from build123d import *

# Parameters (mm, degrees)
SKETCH_1_W          = 57.566503366
SKETCH_1_H          = 9.194649843
EXTRUDE_2_DEPTH     = 9
SKETCH_2_R          = 4.304670881
CUT_EXTRUDE_1_DEPTH = 9
SKETCH_3_R          = 3.25
CUT_EXTRUDE_4_DEPTH = 59.986811199
SKETCH_4_R          = 1.995507564
CUT_EXTRUDE_5_DEPTH = 59.986811199
FILLET_4_R          = 0.2


with BuildPart() as part:
    # 草图1 → 凸台-拉伸2 (new body)
    with BuildSketch(Plane(origin=(0, 0, 0), x_dir=(1, 0, 0), z_dir=(0, 1, 0))):
        with Locations((28.783251683, 4.597324922)):
            Rectangle(SKETCH_1_W, SKETCH_1_H)
    extrude(amount=EXTRUDE_2_DEPTH)

    # 草图2 → 切除-拉伸1 (cut)
    with BuildSketch(Plane(origin=(0, 9, 0), x_dir=(1, 0, 0), z_dir=(0, 1, 0))):
        with Locations(Location((5.562922539, 4.537375707, 0), (0, 0, 270))):
            Circle(SKETCH_2_R)
    extrude(amount=-CUT_EXTRUDE_1_DEPTH, mode=Mode.SUBTRACT)

    # 草图3 → 切除-拉伸4 (cut, through all)
    with BuildSketch(Plane.XY):
        with Locations((25.905689379, 4.639881501)):
            Circle(SKETCH_3_R)
        with Locations((30.901457267, 4.679847644)):
            Circle(SKETCH_3_R)
    extrude(amount=-CUT_EXTRUDE_4_DEPTH, mode=Mode.SUBTRACT)

    # 草图4 → 切除-拉伸5 (cut, through all)
    with BuildSketch(Plane(origin=(0, 9, 0), x_dir=(1, 0, 0), z_dir=(0, 1, 0))):
        with Locations(Location((45.569031787, 4.648915429, 0), (0, 0, 270))):
            Circle(SKETCH_4_R)
        with Locations(Location((53.08266669, 4.648915429, 0), (0, 0, 270))):
            Circle(SKETCH_4_R)
    extrude(amount=-CUT_EXTRUDE_5_DEPTH, mode=Mode.SUBTRACT)

    # 圆角4
    fillet_4_edges = [part.edges().sort_by_distance(p)[0] for p in [
        (5.562922539, 9, -8.842046587),
        (45.569031787, 9, -6.644422993),
        (53.08266669, 9, -6.644422993),
    ]]
    fillet(fillet_4_edges, radius=FILLET_4_R)


solid = part.part
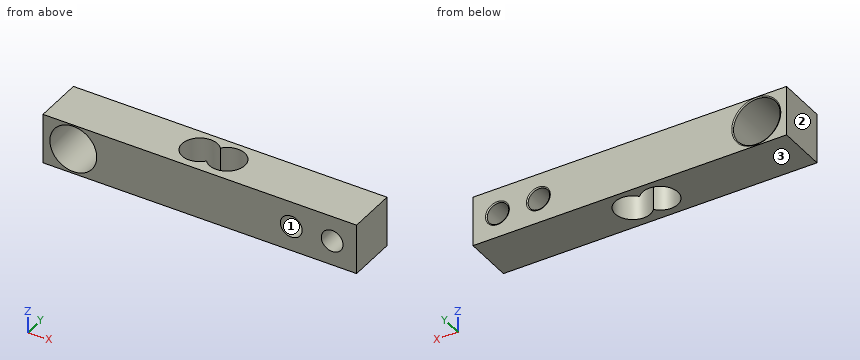
The model under review builds one solid part; all positions refer to its coordinate system, in mm. Face numbers are marked on the shaded views. Coordinates: 2 decimals unless noted, no trailing zeros. Order: outer loops, then holes, each group sorted by start corner. A loop starts at its lowest first (then second) coordinate and runs counter-clockwise, first axis right, second up. Notation, with made-up numbers: (57, 3.25) -> (104, 3.25) arc R13 ccw to (104, 26.25) -> close; hole circle Ø5 at (17, 83.25). An arc over 180 degrees is marked (long way). Answer in a Markdown table with one row per item.
(1) Consider section C-C (z = -5). State how many separate pieces and enclosed holes the cut face has, plus the area to 3 significant figures.
Answers:
| item | result |
|---|---|
| separate pieces | 4 |
| enclosed holes | 1 |
| area | 308 mm² |
(2) Insertion check: pin 1 (3.5 mm diameter, centred on x = 53.08, z = -4.65, fed in from +Y). The pin has a flat end and moves straight along its axis. Give the tip position at first contact, or say it passes through.
Answers:
| item | result |
|---|---|
| pin 1 | through |
(3) Consider section A-A (y = 3.25). Write out the cut boundary in (x, z), plus the area to 3 significant figures.
Answers:
| item | result |
|---|---|
| outline | (0, -9.19) -> (22.97, -9.19) -> (22.97, 0) -> (0, 0) -> close; (33.82, -9.19) -> (57.57, -9.19) -> (57.57, 0) -> (33.82, 0) -> close; hole circle Ø8.61 at (5.56, -4.54); hole circle Ø3.99 at (45.57, -4.65); hole circle Ø3.99 at (53.08, -4.65) |
| area | 346 mm² |
(4) Consider section D-D (y = 6). Write out the cut boundary in (x, z).
Answers:
| item | result |
|---|---|
| outline | (0, -9.19) -> (22.95, -9.19) -> (22.95, 0) -> (0, 0) -> close; (33.87, -9.19) -> (57.57, -9.19) -> (57.57, 0) -> (33.87, 0) -> close; hole circle Ø8.61 at (5.56, -4.54); hole circle Ø3.99 at (45.57, -4.65); hole circle Ø3.99 at (53.08, -4.65) |
(5) Consider section B-B (x = 32.5). Write out the cut boundary in (y, z).
Answers:
| item | result |
|---|---|
| outline | (0, -9.19) -> (1.85, -9.19) -> (1.85, 0) -> (0, 0) -> close; (7.51, -9.19) -> (9, -9.19) -> (9, 0) -> (7.51, 0) -> close |
(6) Wall thickness on line 1 along X through (y, z) = (6.5, -8.5); line 2 along X through (y, z) = (2, -5.75); line 3 along X through (y, z) = (6, -4.5): over which ranges is each line inside the solid? List them lowest first.
Answers:
| item | result |
|---|---|
| line 1 | 0 to 3.88, 7.24 to 23.24, 33.59 to 57.57 |
| line 2 | 0 to 1.43, 9.69 to 24.01, 27.8 to 29.06, 32.74 to 43.9, 47.23 to 51.42, 54.75 to 57.57 |
| line 3 | 0 to 1.26, 9.87 to 22.95, 33.87 to 43.58, 47.56 to 51.09, 55.07 to 57.57 |
(7) The part is to be moulded in two halves that separate along Z. For the marked faces 1, 2 and 3, say which applies: +Z half, -Z half, draft (parallel to the pull), parting line (faces both ways), or undercut.
Answers:
| item | result |
|---|---|
| face 1 | undercut |
| face 2 | draft |
| face 3 | -Z half |
